Work out the finished part from the listing and answer in its coordinate system (mm). A direction names the side the tool comes from. Round coordinates to 2 decimals unless told otherwise and drop trailing zeros. Order: outer loops, then holes, each group sorted by start corner. A loop starts at its lowest first (then second) coordinate and runs counter-clockwise, first axis right, second up. Notation, with made-up numbers: (3, 30.5) -> (36, 30.5) arc R25 ccw to (36, 59.5) -> close; hole circle Ø11 at (-13, 62). An arc over 180 degrees is marked (long way). Use one line per item in the form item = value.
```python
from build123d import *

# Parameters (mm, degrees)
BOSS_EXTRUDE1_DEPTH = 5
BOSS_EXTRUDE2_DEPTH = 1
FILLET1_RADIUS      = 2.5
FILLET1_LENGTH      = 15
FILLET2_RADIUS      = 2.5
FILLET2_LENGTH      = 15
BOSS_EXTRUDE3_START = -6
BOSS_EXTRUDE3_DEPTH = 6
SKETCH5_R           = 1
CUT_EXTRUDE2_DEPTH  = 15


with BuildPart() as part:
    # Sketch2 → Boss-Extrude1 (new body)
    with BuildSketch(Plane.XY):
        with BuildLine():
            Line((-20, 15), (-20, 0))
            Line((-20, 0), (-13.228756555, 0))
            ThreePointArc((-13.228756555, 0), (0, -5), (13.228756555, 0))
            Line((13.228756555, 0), (20, 0))
            Line((20, 0), (20, 15))
            Line((20, 15), (15, 15))
            ThreePointArc((15, 15), (0, 0), (-15, 15))
            Line((-15, 15), (-20, 15))
        make_face()
    extrude(amount=BOSS_EXTRUDE1_DEPTH)

    # Sketch3 → Boss-Extrude2 (add)
    with BuildSketch(Plane.XY.offset(5)):
        with BuildLine():
            Line((-16, 15), (-15, 15))
            ThreePointArc((-15, 15), (0, 0), (15, 15))
            Line((15, 15), (16, 15))
            ThreePointArc((16, 15), (0, -1), (-16, 15))
        make_face()
    extrude(amount=BOSS_EXTRUDE2_DEPTH)

    # Fillet1: full round fillet: the end face becomes a half cylinder, R = half its width
    fillet1_face = Plane((20, 7.5, 2.5), x_dir=(0, -1, 0), z_dir=(1, 0, 0))  # on the end face: x along it, z out of the body
    fillet1_slab = fillet1_face.offset(-FILLET1_RADIUS / 2) * Box(FILLET1_LENGTH, 2 * FILLET1_RADIUS, FILLET1_RADIUS, mode=Mode.PRIVATE)  # the body's end, R deep
    fillet1_round = Plane((17.5, 7.5, 2.5), x_dir=(1, 0, 0), z_dir=(0, -1, 0)) * Cylinder(FILLET1_RADIUS, FILLET1_LENGTH, mode=Mode.PRIVATE)  # its axis R under the face
    add(fillet1_slab - fillet1_round, mode=Mode.SUBTRACT)

    # Fillet2: full round fillet: the end face becomes a half cylinder, R = half its width
    fillet2_face = Plane((-20, 7.5, 2.5), x_dir=(0, -1, 0), z_dir=(-1, 0, 0))  # on the end face: x along it, z out of the body
    fillet2_slab = fillet2_face.offset(-FILLET2_RADIUS / 2) * Box(FILLET2_LENGTH, 2 * FILLET2_RADIUS, FILLET2_RADIUS, mode=Mode.PRIVATE)  # the body's end, R deep
    fillet2_round = Plane((-17.5, 7.5, 2.5), x_dir=(-1, 0, 0), z_dir=(0, -1, 0)) * Cylinder(FILLET2_RADIUS, FILLET2_LENGTH, mode=Mode.PRIVATE)  # its axis R under the face
    add(fillet2_slab - fillet2_round, mode=Mode.SUBTRACT)

    # Sketch3<2> → Boss-Extrude3 (add)
    with BuildSketch(Plane.XY.offset(5).offset(BOSS_EXTRUDE3_START)):
        with BuildLine():
            Line((-16, 15), (-15, 15))
            ThreePointArc((-15, 15), (0, 0), (15, 15))
            Line((15, 15), (16, 15))
            ThreePointArc((16, 15), (0, -1), (-16, 15))
        make_face()
    extrude(amount=BOSS_EXTRUDE3_DEPTH)

    # Sketch5 → Cut-Extrude2 (cut)
    with BuildSketch(Plane(origin=(0, 15, 0), x_dir=(1, 0, 0), z_dir=(0, 1, 0))):
        with Locations(Location((-17, -2.5, 0), (0, 0, 270))):
            Circle(SKETCH5_R)
        with Locations(Location((17, -2.5, 0), (0, 0, 270))):
            Circle(SKETCH5_R)
    extrude(amount=-CUT_EXTRUDE2_DEPTH, mode=Mode.SUBTRACT)


solid = part.part
```
Item 1: The part is cut by section C-C, the plane z = 4. Give the vertices of the cut face in (x, y), and give its area (3 significant figures).
Findings:
outline = (-19.5, 0) -> (-13.23, 0) arc R20 ccw to (13.23, 0) -> (19.5, 0) -> (19.5, 15) -> (15, 15) arc R15 cw to (-15, 15) -> (-19.5, 15) -> close
area = 322 mm^2
Item 2: For faces 1 (the flat face through (15.8, 0, 2.5)), 2 (the flat face through (0, -2, 0)), 3 (the flat face through (0, -2, 5)), determine the directions among +Z, -Z, +X, -X, +Y, -Y from which every point of the face is accessible in a straight line to the end or side of a thin tool.
Findings:
face_1 = +Z, -Z, +X, -Y
face_2 = -Z, -Y
face_3 = +Z, -Y
Item 3: Flat-ended cylindrical pins translate along their axes: P1, Ø3, axis at x = -8, y = -2.5, coming from the +Z side; P2, Ø1.5, axis at x = 17.5, z = 2, coming from the -Y side; P3, Ø10, axis at x = 1.5, y = 7.5, coming from the -Z side. Find the tip coordinate at first contact, or state that the pin passes through.
Findings:
P1 = 5
P2 = 0
P3 = through
Item 4: Determine the mould class of faces 4 (the cylindrical face through (16.024, 7.605, 2.283)), 5 (the cylindrical face through (-20, 7.4, 2.6)), 6 (the flat face through (-15.9, 0, 3)) for opening direction Z: released by +Z, released by -Z, zero draft, split by the parting line, or undercut.
Findings:
face_4 = undercut
face_5 = split by the parting line
face_6 = zero draft
Item 5: The part is cut by section A-A, the plane x = 17. Give the vertices of the cut face in (y, z), and give its area (3 significant figures).
Findings:
outline = (0, 0) -> (15, 0) -> (15, 1.5) -> (0, 1.5) -> close; (0, 3.5) -> (15, 3.5) -> (15, 5) -> (0, 5) -> close
area = 45.0 mm^2
Item 6: The part is cut by section B-B, the plane y = 6.5. Give the vertices of the cut face in (x, z).
Findings:
outline = (-17.5, 0) -> (-13.56, 0) -> (-13.56, -1) -> (-12.36, -1) -> (-12.36, 6) -> (-13.56, 6) -> (-13.56, 5) -> (-17.5, 5) arc R2.5 ccw to start; (12.36, -1) -> (13.56, -1) -> (13.56, 0) -> (17.5, 0) arc R2.5 ccw to (17.5, 5) -> (13.56, 5) -> (13.56, 6) -> (12.36, 6) -> close; hole circle Ø2 at (-17, 2.5); hole circle Ø2 at (17, 2.5)
Item 7: Consider line 1 along X through (y, z) = (6.5, 2.5); line 2 along X through (y, z) = (7, 2.25); line 3 along Z through (x, y) = (4, -1). Determine where each line is inside the solid, lowest interval first.
Findings:
line_1 = -20 to -18, -16 to -12.36, 12.36 to 16, 18 to 20
line_2 = -19.99 to -17.97, -16.03 to -12.69, 12.69 to 16.03, 17.97 to 19.99
line_3 = 0 to 5
Item 8: The part is cut by section D-D, the plane y = 10.5. Give the vertices of the cut face in (x, z).
Findings:
outline = (-17.5, 0) -> (-15.35, 0) -> (-15.35, -1) -> (-14.31, -1) -> (-14.31, 6) -> (-15.35, 6) -> (-15.35, 5) -> (-17.5, 5) arc R2.5 ccw to start; (14.31, -1) -> (15.35, -1) -> (15.35, 0) -> (17.5, 0) arc R2.5 ccw to (17.5, 5) -> (15.35, 5) -> (15.35, 6) -> (14.31, 6) -> close; hole circle Ø2 at (-17, 2.5); hole circle Ø2 at (17, 2.5)
